```python
from build123d import *

# Parameters (mm, degrees)
F0_W     = 20
F0_H     = 20
F1_DEPTH = 20
F2_W     = 7.5
F2_H     = 7.5
F3_DEPTH = 25
F4_W     = 7.5
F4_H     = 7.5
F5_DEPTH = 25
F6_W     = 7.5
F6_H     = 7.5
F7_DEPTH = 25


with BuildPart() as f1:
    # F0 (on Top) → F1 (new body)
    with BuildSketch(Plane.XY):
        with Locations((10, -10)):
            Rectangle(F0_W, F0_H)
    extrude(amount=F1_DEPTH)

    # F2 (on face) → F3 (cut)
    with BuildSketch(Plane.YZ.offset(20)):
        with Locations((-6.25, 13.75)):
            Rectangle(F2_W, F2_H)
        with Locations((-6.25, 6.25)):
            Rectangle(F2_W, F2_H)
        with Locations((-13.75, 6.25)):
            Rectangle(F2_W, F2_H)
        with Locations((-13.75, 13.75)):
            Rectangle(F2_W, F2_H)
    extrude(amount=-F3_DEPTH, mode=Mode.SUBTRACT)

    # F4 (on face) → F5 (cut)
    with BuildSketch(Plane.XY.offset(20)):
        with Locations((13.75, -6.25)):
            Rectangle(F4_W, F4_H)
        with Locations((6.25, -13.75)):
            Rectangle(F4_W, F4_H)
        with Locations((13.75, -13.75)):
            Rectangle(F4_W, F4_H)
        with Locations((6.25, -6.25)):
            Rectangle(F4_W, F4_H)
    extrude(amount=-F5_DEPTH, mode=Mode.SUBTRACT)

    # F6 (on face) → F7 (cut)
    with BuildSketch(Plane(origin=(0, 0, 0), x_dir=(-1, 0, 0), z_dir=(0, 1, 0))):
        with Locations((-13.75, 6.25)):
            Rectangle(F6_W, F6_H)
        with Locations((-6.25, 6.25)):
            Rectangle(F6_W, F6_H)
        with Locations((-13.75, 13.75)):
            Rectangle(F6_W, F6_H)
        with Locations((-6.25, 13.75)):
            Rectangle(F6_W, F6_H)
    extrude(amount=-F7_DEPTH, mode=Mode.SUBTRACT)


solid = f1.part
```
Read the model definition and answer for the solid it produces. Units are mm, in the model's axes. A direction names the side the tool comes from. Give positions to 0.01 mm unless a question says otherwise; leave off trailing zeros. Order: outer loops, then holes, each group sorted by start corner. A loop starts at its lowest first (then second) coordinate and runs counter-clockwise, first axis right, second up.
(1) Find section A-A (y = -9.5). Give the vertices of the cut face in (x, z), plus the area to 3 significant figures.
(2) For faces 4 (the flat face through (19, -2.5, 10)), 5 (the flat face through (2.5, -1, 10)), 6 (the flat face through (10, 0, 19)), 7 (the flat face through (10, -17.5, 1)), determine the directions among +Z, -Z, +X, -X, +Y, -Y from which every point of the face is accessible in a straight line to the end or side of a thin tool.
(3) For a pull along Z with two mould halves and no side action, classify faces 1 (the flat face through (10, -2.5, 1)), 2 (the flat face through (10, -19, 0)), 3 (the flat face through (1, -10, 2.5)) as released by +Z, released by -Z, zero draft, split by the parting line, or undercut.
(4) Straight lines are drawn through the part: L1, parallel to Z at x = 3, y = -19; L2, parallel to Y at x = 9, z = 1. For each, find the intervals that lie inside material, in ascending order.
(5) Find section B-B (z = 17). Give the vertices of the cut face in (x, y).
(6) Find section C-C (y = -2). Give the vertices of the cut face in (x, z), plus the area to 3 significant figures.
Result sheet:
1. outline: (0, 0) - (2.5, 0) - (2.5, 2.5) - (0, 2.5) - close; (0, 17.5) - (2.5, 17.5) - (2.5, 20) - (0, 20) - close; (17.5, 0) - (20, 0) - (20, 2.5) - (17.5, 2.5) - close; (17.5, 17.5) - (20, 17.5) - (20, 20) - (17.5, 20) - close
1. area: 25.0 mm2
2. face 4: +X, -X
2. face 5: +Y, -Y
2. face 6: +Z, -Z, +X, -X, +Y
2. face 7: +Z, -Z
3. face 1: zero draft
3. face 2: released by -Z
3. face 3: undercut
4. L1: z = 0 to 2.5, 17.5 to 20
4. L2: y = -20 to -17.5, -2.5 to 0
5. outline: (0, -20) - (2.5, -20) - (2.5, -17.5) - (0, -17.5) - close; (0, -2.5) - (2.5, -2.5) - (2.5, 0) - (0, 0) - close; (17.5, -20) - (20, -20) - (20, -17.5) - (17.5, -17.5) - close; (17.5, -2.5) - (20, -2.5) - (20, 0) - (17.5, 0) - close
6. outline: (0, 0) - (20, 0) - (20, 20) - (0, 20) - close; hole (2.5, 2.5) - (17.5, 2.5) - (17.5, 17.5) - (2.5, 17.5) - close
6. area: 175 mm2
